The drawing under review shows one solid part. Ordinate dimensions are in mm from its lowest x, y, z. A direction names the side the tool comes from. Round coordinates to 2 decimals unless told otherwise and drop trailing zeros. Order: outer loops, then holes, each group sorted by start corner. A loop starts at its lowest first (then second) coordinate and runs counter-clockwise, first axis right, second up. Notation, with made-up numbers: (-1.75, 23.25) -> (8.25, 23.25) arc R22 ccw to (8.25, 35.25) -> close; hole circle Ø7 at (-22, -26.75). An arc over 180 degrees is marked (long way). Use a Markdown table: item, result. Add a question column.
1) Consider section B-B (x = 5). State the section outline as (y, z) points, plus the area to 3 significant figures.
2) Clearance check with flat-ended pins moving along their axes: P1, Ø3, axis at x = 6.5, z = 10, coming from the -Y side; P2, Ø1.5, axis at x = 3.5, y = 13, coming from the -Z side; P3, Ø5, axis at x = 5.5, z = 6.5, coming from the +Y side; P4, Ø2.5, axis at x = 5, y = 10, coming from the -Z side. State where each tip first meets the part, or that it passes through.
3) Consider section A-A (z = 5). State the section outline as (x, y) points, plus the area to 3 significant figures.
4) Consider section D-D (z = 11.25). State the section outline as (x, y) points.
5) Consider section C-C (y = 9.75). State the section outline as (x, z) points, plus the area to 3 significant figures.
6) Machinability: for the marked faces 4 and 5, which of the approach directions +Z, -Z, +X, -X, +Y, -Y give a long, thin tool a straight path to every point of the face, cutting with its end or side? Answer none if there is none.
7) Draft analysis for pull direction Z (two halves, no side actions). For the marked faces 1, 2 and 3, state which applies: pulls with the +Z half, pulls with the -Z half, needs draft (parallel to the pull), parting line crosses it, or undercut.
8) Wall thickness on line 1 along Z through (x, y) = (5, 2.35); line 2 along Y through (x, z) = (5, 11.35); line 3 along X through (y, z) = (3.15, 5): over which ranges is each line inside the solid? List them lowest first. Write a range as [from, to].
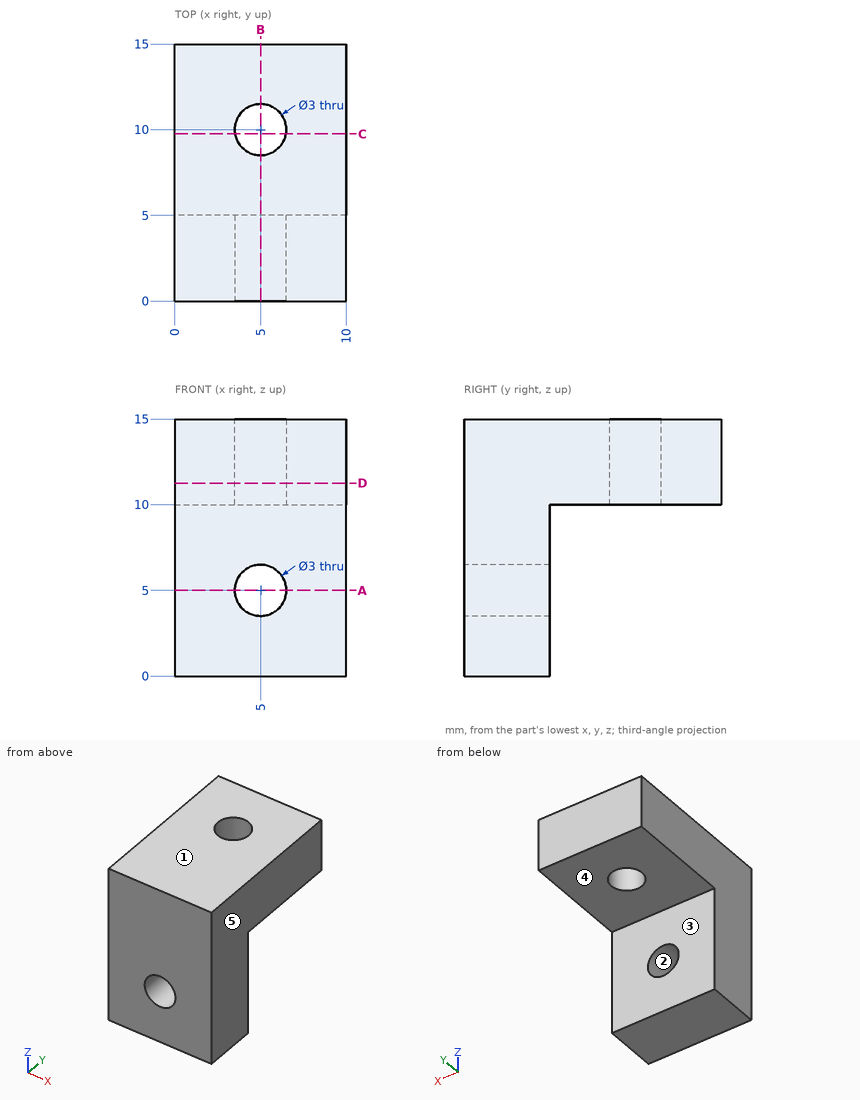
Results list:
| question | item | result |
|---|---|---|
| 1 | outline | (0, 0) -> (5, 0) -> (5, 3.5) -> (0, 3.5) -> close; (0, 6.5) -> (5, 6.5) -> (5, 10) -> (8.5, 10) -> (8.5, 15) -> (0, 15) -> close; (11.5, 10) -> (15, 10) -> (15, 15) -> (11.5, 15) -> close |
| 1 | area | 95.0 mm2 |
| 2 | P1 | y = 0 |
| 2 | P2 | z = 10 |
| 2 | P3 | y = 5 |
| 2 | P4 | through |
| 3 | outline | (0, 0) -> (3.5, 0) -> (3.5, 5) -> (0, 5) -> close; (6.5, 0) -> (10, 0) -> (10, 5) -> (6.5, 5) -> close |
| 3 | area | 35.0 mm2 |
| 4 | outline | (0, 0) -> (10, 0) -> (10, 15) -> (0, 15) -> close; hole circle Ø3 at (5, 10) |
| 5 | outline | (0, 10) -> (3.52, 10) -> (3.52, 15) -> (0, 15) -> close; (6.48, 10) -> (10, 10) -> (10, 15) -> (6.48, 15) -> close |
| 5 | area | 35.2 mm2 |
| 6 | face 4 | -Z, +X, -X, +Y |
| 6 | face 5 | +Z, -Z, +X, +Y, -Y |
| 7 | face 1 | pulls with the +Z half |
| 7 | face 2 | undercut |
| 7 | face 3 | needs draft |
| 8 | line 1 | [0, 3.5], [6.5, 15] |
| 8 | line 2 | [0, 8.5], [11.5, 15] |
| 8 | line 3 | [0, 3.5], [6.5, 10] |
